Check sheet for the modelled part. Datum: model origin and axes. Units: mm. Give positions to 0.01 mm unless a question says otherwise; leave off trailing zeros. Loops run counter-clockwise (first coordinate to the right, second up) from the corner with the lowest first, then second, coordinate; pieces in that order, holes last. Notation, with made-up numbers: (55, 46.25) -> (107, 46.25) arc R35 ccw to (107, 78.25) -> close; hole circle Ø2 at (60, 29.25). An arc over 180 degrees is marked (long way). Write each question's results on one line, items separated by ' | '. Start each with the question number.
Item 1: Gauge pin test, flat end, axial feed: pin 1 Ø4 at (x, y) = (-10, 77) entering from +Z. Record the tip position at first contact, or that the pin passes through.
Item 2: Cross-section at A-A on x = 0. Enter the section's corners in (y, z), then the cut area to 3 significant figures.
Item 3: Scan lines: line 1 along Y through (x, z) = (0.5, 6.5); line 2 along Z through (x, y) = (-12, -296); line 3 along Y through (x, z) = (4, 7.5). Record each from-to range of solid material in increasing order.
Item 4: Cross-section at B-B on y = -325. Enter the section's corners in (x, z).
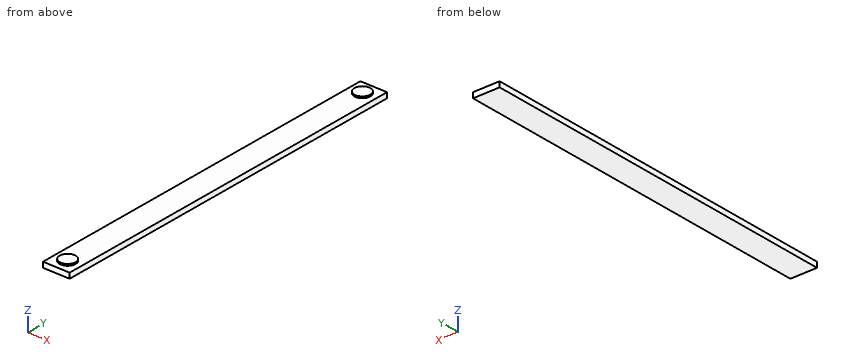
from build123d import *

# Parameters (mm, degrees)
SKETCH1_W           = 50
SKETCH1_H           = 700
BOSS_EXTRUDE1_DEPTH = 5
SKETCH2_R           = 15
BOSS_EXTRUDE2_DEPTH = 3


with BuildPart() as part:
    # Sketch1 → Boss-Extrude1 (new, symmetric)
    with BuildSketch(Plane.XY):
        Rectangle(SKETCH1_W, SKETCH1_H)
    extrude(amount=BOSS_EXTRUDE1_DEPTH, both=True)

    # Sketch2 → Boss-Extrude2 (add)
    with BuildSketch(Plane.XY.offset(5)):
        with Locations((0, -325)):
            Circle(SKETCH2_R)
        with Locations((0, 325)):
            Circle(SKETCH2_R)
    extrude(amount=BOSS_EXTRUDE2_DEPTH)


solid = part.part
Answer sheet:
1) pin 1: stops at z = 5
2) outline: (-350, -5) -> (350, -5) -> (350, 5) -> (340, 5) -> (340, 8) -> (310, 8) -> (310, 5) -> (-310, 5) -> (-310, 8) -> (-340, 8) -> (-340, 5) -> (-350, 5) -> close | area: 7,180 mm²
3) line 1: y = -339.99 to -310.01, 310.01 to 339.99 | line 2: z = -5 to 5 | line 3: y = -339.46 to -310.54, 310.54 to 339.46
4) outline: (-25, -5) -> (25, -5) -> (25, 5) -> (15, 5) -> (15, 8) -> (-15, 8) -> (-15, 5) -> (-25, 5) -> close
